Model file for the job. Use its own axes, mm. A direction names the side the tool comes from. Round coordinates to 2 decimals unless told otherwise and drop trailing zeros. Loops run counter-clockwise (first coordinate to the right, second up) from the corner with the lowest first, then second, coordinate; pieces in that order, holes last. Notation, with made-up numbers: (-32, 38) -> (-3, 38) arc R7 ccw to (-3, 47) -> close; hole circle Ø11 at (72.5, 24). An arc over 180 degrees is marked (long way). Use a Markdown table: item, result.
from build123d import *

# Parameters (mm, degrees)
F0_R     = 6.5
F0_R_2   = 0.9
F1_DEPTH = 2
F2_SIZE  = 1.99999
F3_R     = 6.5
F4_DEPTH = 2.7


# Not quite as in the source:
# - a fillet or chamfer is up to 0.001 mm smaller than in the source, because OpenCascade refuses the exact size


with BuildPart() as f1:
    # F0 (on Top) → F1 (new body)
    with BuildSketch(Plane.XY):
        Circle(F0_R)
        Circle(F0_R_2, mode=Mode.SUBTRACT)
    extrude(amount=F1_DEPTH)

    # F2 (size 2 in the source; OpenCascade refuses exactly that, so slightly less here)
    f2_edges = [f1.edges().sort_by_distance(p)[0] for p in [
        (-0.9, 0, 2),
    ]]
    chamfer(f2_edges, length=F2_SIZE)

    # F3 (on face) → F4 (join)
    with BuildSketch(Plane.XY.offset(2)):
        Circle(F3_R)
        Polygon((-2.8920572149, 2.9859680282), (1.1398955598, 3.9975790314), (4.0319527748, 1.0116110032), (2.8920572149, -2.9859680282), (-1.1398955598, -3.9975790314), (-4.0319527748, -1.0116110032), align=None, mode=Mode.SUBTRACT)
    extrude(amount=F4_DEPTH)


solid = f1.part
Q1. Band-saw the part on A-A, the plane z = 3.05. Give the cut face in (x, y), plus the area to 3 significant figures.
Results list:
| item | result |
|---|---|
| outline | circle Ø13 at (0, 0); hole (-4.03, -1.01) -> (-1.14, -4) -> (2.89, -2.99) -> (4.03, 1.01) -> (1.14, 4) -> (-2.89, 2.99) -> close |
| area | 87.8 mm² |
Q2. Flat gauge pins, fed straight in: pin 1 (1 mm diameter, centred on x = 1.5, y = 2, fed in from +Z); pin 2 (2.5 mm diameter, centred on x = -1.5, y = -0.5, fed in from +Z); pin 3 (1.5 mm diameter, centred on y = -4, z = 0.5, fed in from +X). Where does each tip first touch, or does it go through?
Results list:
| item | result |
|---|---|
| pin 1 | stops at z = 2 |
| pin 2 | stops at z = 1.93 |
| pin 3 | stops at x = 5.63 |
Q3. Pull direction Y, two halves, no side cores. Call faces 3 (the face through (1, -3, 2)), 4 (the face through (-5.158, -3.955, 2.317)), 5 (the face through (3.47, -0.96, 3.33)), 6 (the face through (3, 3, 4.7)): released by +Y, released by -Y, zero draft, split by the parting line, or undercut.
Results list:
| item | result |
|---|---|
| face 3 | undercut |
| face 4 | split by the parting line |
| face 5 | undercut |
| face 6 | zero draft |
Q4. Band-saw the part on D-D, the plane y = -3.75. Give the cut face in (x, z).
Results list:
| item | result |
|---|---|
| outline | (-5.31, 0) -> (5.31, 0) -> (5.31, 4.7) -> (-0.15, 4.7) -> (-0.15, 2) -> (-1.38, 2) -> (-1.38, 4.7) -> (-5.31, 4.7) -> close |
Q5. Drill centre lines: L1, parallel to Z at x = 2, y = -3; L2, parallel to Y at x = 0, z = 0.05; L3, parallel to Y at x = 1.25, z = 1.65. Where is each one in solid material? Low to high. Write a range as from..to.
Results list:
| item | result |
|---|---|
| L1 | z = 0..2 |
| L2 | y = -6.5..-0.95, 0.95..6.5 |
| L3 | y = -6.38..-2.22, 2.22..6.38 |
Q6. Tool access for faces 1 (the face through (1.4, 0.1, 0)), 2 (the face through (2.566, 2.525, 3.331)): list every direction of +Z, -Z, +X, -X, +Y, -Y with a clear straight run to the whole face (end or side of a thin tool).
Results list:
| item | result |
|---|---|
| face 1 | -Z, +X, -X, +Y, -Y |
| face 2 | +Z |
